CAD build for the part. Positions are in the model's coordinates, mm. A direction names the side the tool comes from. Coordinates: 2 decimals unless noted, no trailing zeros. Use one line per item in the form item = value.
Autodesk Inventor part; units mm, degrees
ref_plane "Pracovní rovina4" through (0, 0, 0) normal (1, 0, 0) x (0, 1, 0)
ref_plane "XZ Plane" through (0, 0, 0) normal (0, 1, 0) x (-1, 0, 0)
ref_plane "XY Plane" through (0, 0, 0) normal (0, 0, 1) x (1, 0, 0)
sketch "Náčrt1" plane through (0, 0, 0) normal (0, 0, 1) x (1, 0, 0)
  line L0 (25, -35) -> (-25, 35) construction
  line L1 (-25, -35) -> (25, 35) construction
  arc A0 (-20.9313, 37.9062) -> (-29.0687, 32.0938) centre (-25, 35) ccw
  arc A1 (29.0687, 32.0938) -> (20.9313, 37.9062) centre (25, 35) ccw
  arc A2 (-29.0687, -32.0938) -> (-20.9313, -37.9062) centre (-25, -35) ccw
  arc A3 (20.9313, -37.9062) -> (29.0687, -32.0938) centre (25, -35) ccw
  line L2 (20.9313, 37.9062) -> (0, 8.6023)
  line L3 (-6.1445, 0) -> (-29.0687, -32.0938)
  line L4 (29.0687, -32.0938) -> (6.1445, 0)
  line L5 (0, 8.6023) -> (-20.9313, 37.9062)
  line L6 (-20.9313, -37.9062) -> (0, -8.6023)
  line L7 (6.1445, 0) -> (29.0687, 32.0938)
  line L8 (-29.0687, 32.0938) -> (-6.1445, 0)
  line L9 (0, -8.6023) -> (20.9313, -37.9062)
  line L10 (-44.7648, 0) -> (44.7648, 0)
  line L11 (0, 58.7648) -> (0, -58.7648)
  point P0 (0, 0)
  dimension "d2" = 50
  dimension "d3" = 70
  dimension "d7" = 10
  dimension "d8" = 10
  dimension "d9" = 10
  dimension "d10" = 10
  dimension "d56" = 71.075
  dimension "d57" = 108.925
extrude "Vysunutí1" add sketch "Náčrt1" along normal mid plane 10
fillet "Zaoblení1" radius 10 4 edges at (6.1445, 0, 0) (-6.1445, 0, 0) (0, 8.6023, 0) (0, -8.6023, 0)
ref_plane "Pracovní rovina4" through (0, 0, 0) normal (1, 0, 0) x (0, 1, 0)
sketch "Náčrt4" plane through (0, 0, 0) normal (1, 0, 0) x (0, 1, 0)
  line L0 (-35, 0) -> (35, 0)
  line L1 (0, 35) -> (0, -35)
  point P0 (0, 0)
  point P1 (25, 0)
  point P2 (-25, 0)
hole "Díra1" at (0, 25, 0) at (0, -25, 0) direction (-1, 0, 0) diameter 6 end through all both
fillet "Zaoblení3" radius 2 12 edges at (-19.6824, 18.9531, -5) (-27.9062, 39.0687, -5) (-14.5343, 28.9504, -5) (14.5343, 28.9504, -5) (27.9062, 39.0687, -5) (19.6824, 18.9531, -5) (19.6824, -18.9531, -5) (27.9062, -39.0687, -5) (14.5343, -28.9504, -5) (-14.5343, -28.9504, -5) (-27.9062, -39.0687, -5) (-19.6824, -18.9531, -5)
ref_plane "Pracovní rovina5" through (-25, -35, -3) normal (-0.8137, 0.5812, 0) x (0, 0, 1)
properties part number "vetrovaniig"
Item 1: Drop flat-ended pins along their axis: pin 1 (2 mm diameter, centred on y = 19.5, z = -4, fed in from -X); pin 2 (4 mm diameter, centred on x = -6.5, z = -1, fed in from +Y); pin 3 (2 mm diameter, centred on x = -6, z = 1.5, fed in from +Y); pin 4 (2 mm diameter, centred on x = -24, z = -2.5, fed in from +Y). Give the stop position or say it passes through.
Derived:
pin_1 = -20.62
pin_2 = 20.5
pin_3 = 18.67
pin_4 = 40
Item 2: Cut at A-A, the plane z = 0. State how many separate pieces and enclosed holes the cut face has, plus the area to 3 significant figures.
Derived:
separate_pieces = 5
enclosed_holes = 0
area = 1,590 mm²
Item 3: Two-plate mould, pull along Y, no slides. Class faces 1 (the face through (-16, 31, 1)), 2 (the face through (0, 0, -5)), 3 (the face through (19.087, -19.101, -4.399)): +Y half, -Y half, draft (parallel to the pull), parting line (faces both ways), or undercut.
Derived:
face_1 = +Y half
face_2 = draft
face_3 = undercut
Item 4: 3-axis set-ups, long thin cutter, end or side, ignore diameter. For faces 4 (the face through (16, -31, 1)), 5 (the face through (16, 31, 1)), 6 (the face through (-19.087, 19.101, -4.399)): which of +Z, -Z, +X, -X, +Y, -Y reach the whole face in a straight line?
Derived:
face_4 = +Z, -Z, -Y
face_5 = +Z, -Z, +Y
face_6 = -Z, -X
Item 5: Drill centre lines: line 1 (Y direction, x = 14, z = 0); line 2 (Y direction, x = -17, z = -2); line 3 (X direction, y = 33.5, z = 4). Where is each one in solid material? Low to high. Write a range as [from, to].
Derived:
line_1 = [-28.2, -28], [-22, -11], [11, 22], [28, 28.2]
line_2 = [-32.4, -27.24], [-22.76, -15.2], [15.2, 22.76], [27.24, 32.4]
line_3 = [-29.77, -17.78], [17.78, 29.77]
